The model under review builds one solid part; all positions refer to its coordinate system, in mm. Coordinates: 2 decimals unless noted, no trailing zeros. Write each loop counter-clockwise with the first axis right and the second up, starting at its lowest first coordinate (ties: lowest second). Pieces come first, ordered by that corner, then holes. Notation, with made-up numbers: (71.5, -15.5) - (83.5, -15.5) arc R19 cw to (83.5, 12.5) - close; hole circle Ø5 at (47.25, 27.25). An arc over 180 degrees is marked (long way). Answer as CSV lines item,"result". Start each with the question number.
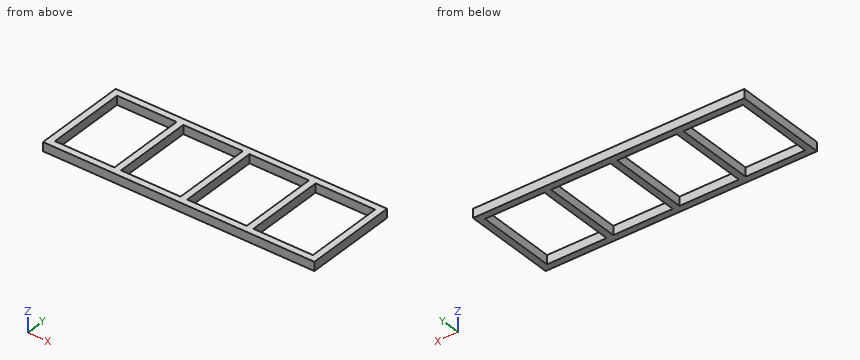
```python
from build123d import *

# Parameters (mm, degrees)
F0_W     = 1549.4
F0_H     = 38.1
F1_DEPTH = 50.8
F2_W     = 38.1
F2_H     = 457.2
F3_DEPTH = 50.8


with BuildPart() as f1:
    # F0 (on Top) → F1 (new body)
    with BuildSketch(Plane.XY):
        with Locations((0, 234.95)):
            Rectangle(F0_W, F0_H)
        with Locations((0, -260.35)):
            Rectangle(F0_W, F0_H)
    extrude(amount=F1_DEPTH)

    # F2 (on Top) → F3 (join, through all)
    with BuildSketch(Plane.XY):
        with Locations((-755.65, -12.7)):
            Rectangle(F2_W, F2_H)
        with Locations((-377.825, -12.7)):
            Rectangle(F2_W, F2_H)
        with Locations((0, -12.7)):
            Rectangle(F2_W, F2_H)
        with Locations((377.825, -12.7)):
            Rectangle(F2_W, F2_H)
        with Locations((755.65, -12.7)):
            Rectangle(F2_W, F2_H)
    extrude(amount=F3_DEPTH)


solid = f1.part
```
(1) Add section A-A on y = 91. Give the boundary of the cut face in (x, z) (3 decimals), then the cut area to 3 significant figures.
(2) Add section B-B on x = 272. Give the boundary of the cut face in (y, z), then the cut area to 3 significant figures.
(3) Add section C-C on z = 33.5. Give the boundary of the cut face in (x, y) (3 decimals), then the cut area to 3 significant figures.
(4) Wall thickness on line 1 (X direction, y = -89.5, z = 27.5) (3 decimals); line 2 (Y direction, x = 490, z = 48.5): over which ranges is each line inside the solid? List them lowest first.
(5) For pin 1 (12 mm diameter, centred on x = 399, y = -212.5, fed in from +Z), flat-tipped, find the tip position at first contact; note if it passes through.
Reported:
1,outline,"(-774.7, 0) - (-736.6, 0) - (-736.6, 50.8) - (-774.7, 50.8) - close; (-396.875, 0) - (-358.775, 0) - (-358.775, 50.8) - (-396.875, 50.8) - close; (-19.05, 0) - (19.05, 0) - (19.05, 50.8) - (-19.05, 50.8) - close; (358.775, 0) - (396.875, 0) - (396.875, 50.8) - (358.775, 50.8) - close; (736.6, 0) - (774.7, 0) - (774.7, 50.8) - (736.6, 50.8) - close"
1,area,"9,680 mm²"
2,outline,"(-279.4, 0) - (-241.3, 0) - (-241.3, 50.8) - (-279.4, 50.8) - close; (215.9, 0) - (254, 0) - (254, 50.8) - (215.9, 50.8) - close"
2,area,"3,870 mm²"
3,outline,"(-774.7, -279.4) - (774.7, -279.4) - (774.7, 254) - (-774.7, 254) - close; hole (-736.6, -241.3) - (-396.875, -241.3) - (-396.875, 215.9) - (-736.6, 215.9) - close; hole (-358.775, -241.3) - (-19.05, -241.3) - (-19.05, 215.9) - (-358.775, 215.9) - close; hole (19.05, -241.3) - (358.775, -241.3) - (358.775, 215.9) - (19.05, 215.9) - close; hole (396.875, -241.3) - (736.6, -241.3) - (736.6, 215.9) - (396.875, 215.9) - close"
3,area,"205,000 mm²"
4,line 1,"-774.7 to -736.6, -396.875 to -358.775, -19.05 to 19.05, 358.775 to 396.875, 736.6 to 774.7"
4,line 2,"-279.4 to -241.3, 215.9 to 254"
5,pin 1,"z = 50.8"
